Design review of the part shown in the three views and the two pictorial views. Dimensions are in mm from the part's minimum x, y and z. A direction names the side the tool comes from. Give positions to 0.01 mm unless a question says otherwise; leave off trailing zeros. Order: outer loops, then holes, each group sorted by start corner. A loop starts at its lowest first (then second) coordinate and runs counter-clockwise, first axis right, second up.
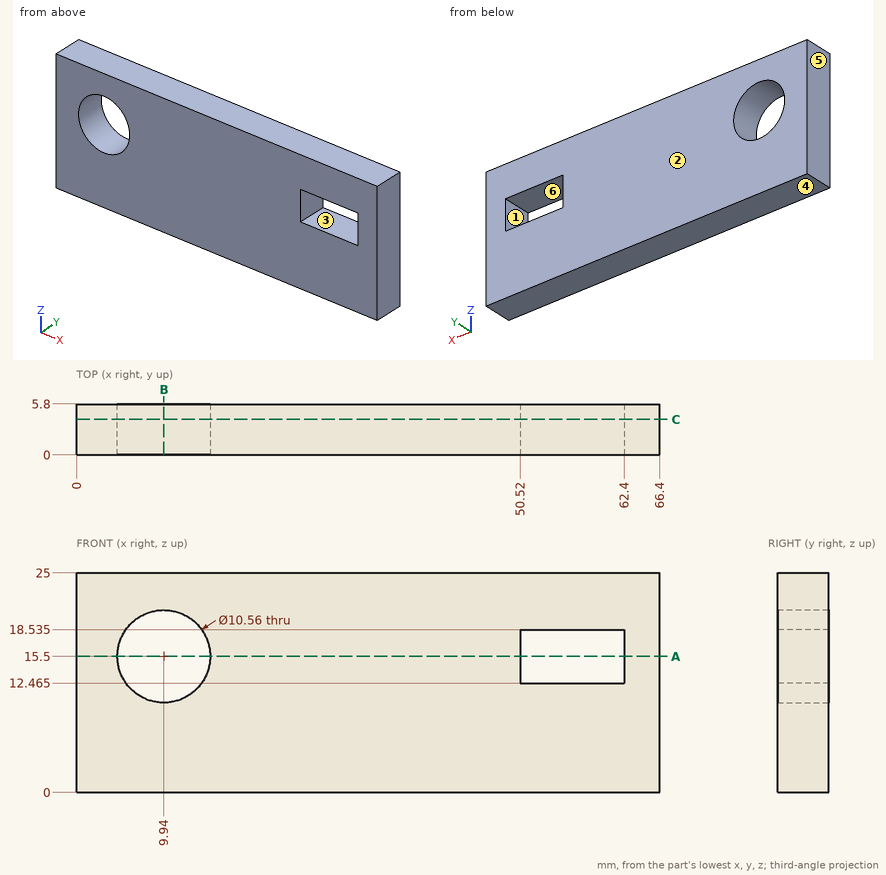
1) Clearance check with a flat-ended pin moving along its axis: pin 1 (10 mm diameter, centred on x = 39, z = 22, fed in from -Y). State where the tip first meets the part, or that it passes through.
Answer sheet:
pin 1: stops at y = 0
2) We need section C-C on y = 4.05. Give the boundary of the cut face in (x, z) (3 decimals), then the cut area to 3 significant figures.
Answer sheet:
outline: (0, 0) - (66.4, 0) - (66.4, 25) - (0, 25) - close; hole circle Ø10.56 at (9.94, 15.5); hole (50.52, 12.465) - (62.4, 12.465) - (62.4, 18.535) - (50.52, 18.535) - close
area: 1,500 mm2
3) To check wall thickness, follow line 1 (X direction, y = 4.3, z = 15.25); line 2 (Z direction, x = 54.5, y = 4.7) (3 decimals); line 3 (Z direction, x = 9.94, y = 3.8). State the ranges of each line that lie inside material, in increasing order.
Answer sheet:
line 1: x = 0 to 4.67, 15.21 to 50.52, 62.4 to 66.4
line 2: z = 0 to 12.465, 18.535 to 25
line 3: z = 0 to 10.22, 20.78 to 25
4) We need section B-B on x = 9.94. Give the boundary of the cut face in (y, z), then the cut area to 3 significant figures.
Answer sheet:
outline: (0, 0) - (5.8, 0) - (5.8, 10.22) - (0, 10.22) - close; (0, 20.78) - (5.8, 20.78) - (5.8, 25) - (0, 25) - close
area: 83.8 mm2
5) Tool access review of the marked faces 1 and 2: name each direction out of +Z, -Z, +X, -X, +Y, -Y from which nothing blocks a thin tool from reaching the whole face with its end or side.
Answer sheet:
face 1: +Y, -Y
face 2: +Z, -Z, +X, -X, +Y
6) We need section A-A on z = 15.5. Give the boundary of the cut face in (x, y).
Answer sheet:
outline: (0, 0) - (4.66, 0) - (4.66, 5.8) - (0, 5.8) - close; (15.22, 0) - (50.52, 0) - (50.52, 5.8) - (15.22, 5.8) - close; (62.4, 0) - (66.4, 0) - (66.4, 5.8) - (62.4, 5.8) - close
7) Draft analysis for pull direction X (two halves, no side actions). For the marked faces 3, 4, 5 and 6, state which applies: +X half, -X half, draft (parallel to the pull), parting line (faces both ways), or undercut.
Answer sheet:
face 3: undercut
face 4: draft
face 5: -X half
face 6: undercut
